Design review of the part shown in the three views and the two pictorial views. Dimensions are in mm from the part's minimum x, y and z. A direction names the side the tool comes from. Coordinates: 2 decimals unless noted, no trailing zeros. Loops run counter-clockwise (first coordinate to the right, second up) from the corner with the lowest first, then second, coordinate; pieces in that order, holes last. Notation, with made-up numbers: (9, 8) -> (52, 8) arc R32 ccw to (52, 47) -> close; hole circle Ø11 at (21.5, -1.75). An arc over 180 degrees is marked (long way). Use CSV: the item, a comma, the result in double quotes.
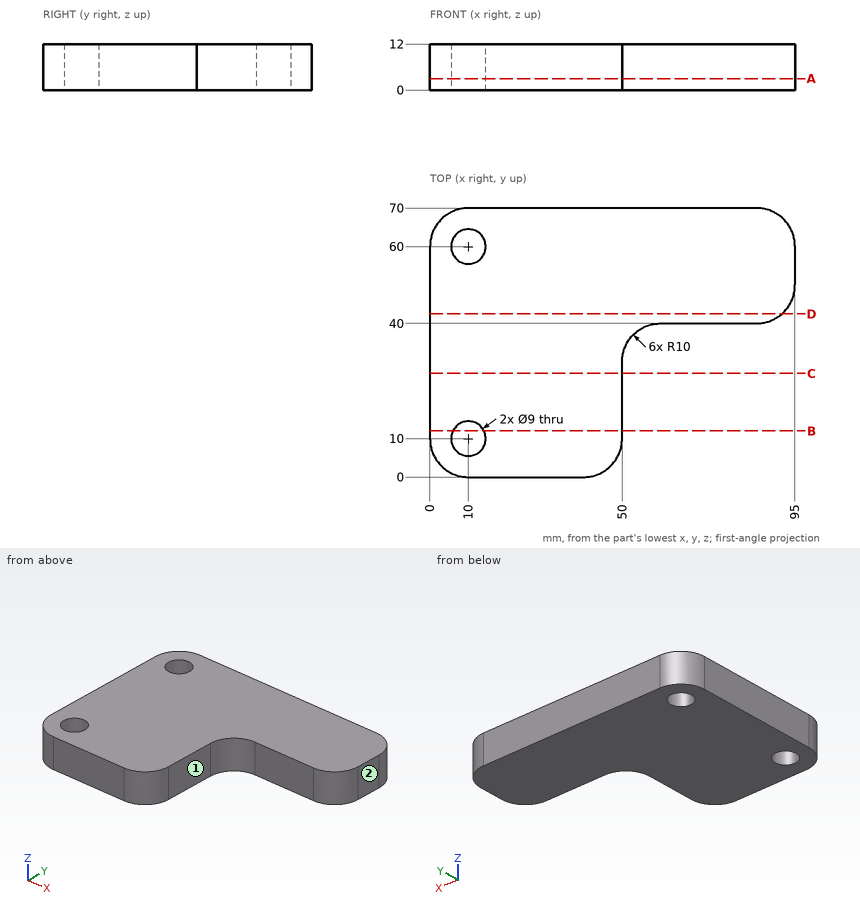
Item 1: Add section B-B (y = 12). Give the boundary of the cut face in (x, z), then the cut area to 3 significant figures.
Checked values:
outline,"(0, 0) -> (5.97, 0) -> (5.97, 12) -> (0, 12) -> close; (14.03, 0) -> (50, 0) -> (50, 12) -> (14.03, 12) -> close"
area,"503 mm^2"
Item 2: Add section C-C (y = 27). Give the boundary of the cut face in (x, z).
Checked values:
outline,"(0, 0) -> (50, 0) -> (50, 12) -> (0, 12) -> close"
Item 3: Add section D-D (y = 42.5). Give the boundary of the cut face in (x, z), then the cut area to 3 significant figures.
Checked values:
outline,"(0, 0) -> (91.61, 0) -> (91.61, 12) -> (0, 12) -> close"
area,"1,100 mm^2"
Item 4: Add section A-A (z = 3). Give the boundary of the cut face in (x, y).
Checked values:
outline,"(0, 10) arc R10 ccw to (10, 0) -> (40, 0) arc R10 ccw to (50, 10) -> (50, 30) arc R10 cw to (60, 40) -> (85, 40) arc R10 ccw to (95, 50) -> (95, 60) arc R10 ccw to (85, 70) -> (10, 70) arc R10 ccw to (0, 60) -> close; hole circle Ø9 at (10, 10); hole circle Ø9 at (10, 60)"
Item 5: Machinability: for the marked faces 1 and 2, which of the approach directions +Z, -Z, +X, -X, +Y, -Y give a long, thin tool a straight path to every point of the face, cutting with its end or side? Answer none if there is none.
Checked values:
face 1,"+Z, -Z, +X, -Y"
face 2,"+Z, -Z, +X, +Y, -Y"
Item 6: Clearance check with flat-ended pins moving along their axes: pin 1 (3 mm diameter, centred on y = 15.5, z = 3, fed in from +X); pin 2 (5.5 mm diameter, centred on x = 10, y = 10, fed in from +Z); pin 3 (3 mm diameter, centred on y = 40.5, z = 8.5, fed in from +X); pin 4 (1 mm diameter, centred on x = 57.5, z = 8, fed in from -Y). State where each tip first meets the part, or that it passes through.
Checked values:
pin 1,"x = 50"
pin 2,"through"
pin 3,"x = 91"
pin 4,"y = 39.54"
Item 7: To check wall thickness, follow line 1 along Y through (x, z) = (10.5, 7.25); line 2 along Y through (x, z) = (63, 8.5); line 3 along X through (y, z) = (22, 9.5). State the ranges of each line that lie inside material, in increasing order.
Checked values:
line 1,"0 to 5.53, 14.47 to 55.53, 64.47 to 70"
line 2,"40 to 70"
line 3,"0 to 50"
